Verification items for this drawing (mm, ordinates from the low corner). Round coordinates to 2 decimals unless told otherwise and drop trailing zeros. Write each loop counter-clockwise with the first axis right and the second up, starting at its lowest first coordinate (ties: lowest second). Pieces come first, ordered by that corner, then holes.
Item 1: Cross-section at C-C (z = 12.7). Enter the section's corners in (x, y).
Item 2: Scan lines: probe 1 along X at (y, z) = (2.85, 12.7); probe 2 along Z at (x, y) = (38.1, 3.1); probe 3 along X at (y, z) = (2.9, 23.25). Record each from-to range of solid material in increasing order.
Item 3: Cross-section at B-B (y = 3.25). Enter the section's corners in (x, z).
Item 4: Depth check by flat-ended pin: P1, Ø7.5, axis at x = 38.1, z = 12.7, coming from the -Y side; P2, Ø2.5, axis at y = 2.5, z = 1.5, coming from the +X side. Enter the tip coordinate at first touch or a pass-through.
Item 5: Cross-section at D-D (z = 23.75). Enter the section's corners in (x, y), then the cut area to 3 significant figures.
Item 6: Cross-section at A-A (x = 38.1). Enter the section's corners in (y, z), then the cut area to 3 significant figures.
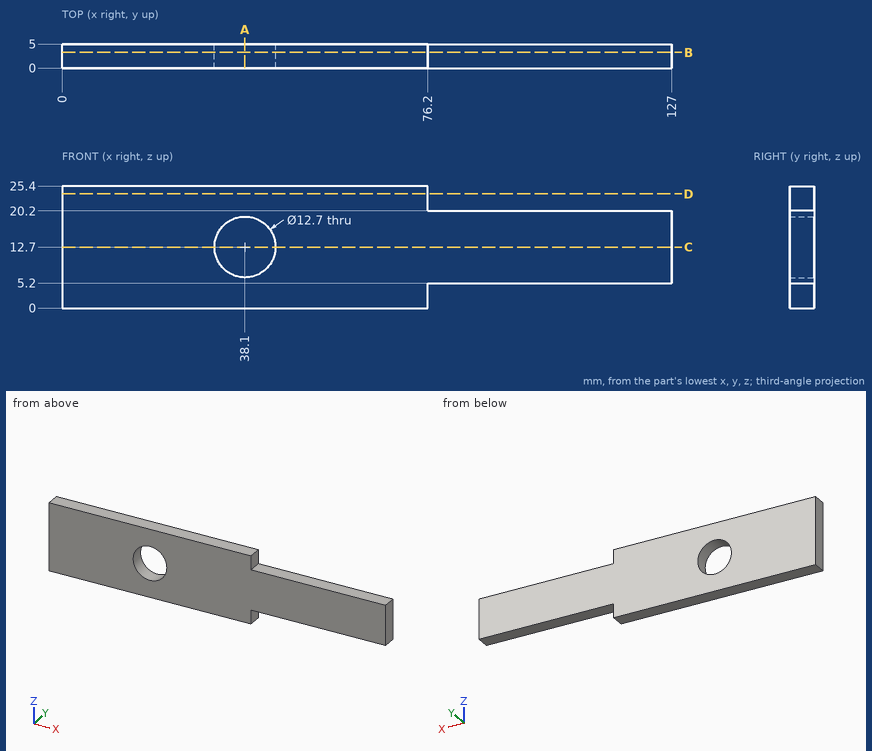
Resolved:
1. outline: (0, 0) - (31.75, 0) - (31.75, 5) - (0, 5) - close; (44.45, 0) - (127, 0) - (127, 5) - (44.45, 5) - close
2. probe 1: x = 0 to 31.75, 44.45 to 127
2. probe 2: z = 0 to 6.35, 19.05 to 25.4
2. probe 3: x = 0 to 76.2
3. outline: (0, 0) - (76.2, 0) - (76.2, 5.2) - (127, 5.2) - (127, 20.2) - (76.2, 20.2) - (76.2, 25.4) - (0, 25.4) - close; hole circle Ø12.7 at (38.1, 12.7)
4. P1: passes through
4. P2: stops at x = 76.2
5. outline: (0, 0) - (76.2, 0) - (76.2, 5) - (0, 5) - close
5. area: 381 mm2
6. outline: (0, 0) - (5, 0) - (5, 6.35) - (0, 6.35) - close; (0, 19.05) - (5, 19.05) - (5, 25.4) - (0, 25.4) - close
6. area: 63.5 mm2
